Part print with two shaded views. Sizes in mm from the minimum x, y, z corner. A direction names the side the tool comes from. Round coordinates to 2 decimals unless told otherwise and drop trailing zeros. Order: outer loops, then holes, each group sorted by start corner. A loop starts at its lowest first (then second) coordinate and runs counter-clockwise, first axis right, second up. Notation, with made-up numbers: M -17,-24 L 34,-24 A30 ccw 34,13 Z; hole C 15.5,-22.75 d2. An arc over 180 degrees is marked long. Put each result on its own line as item: value.
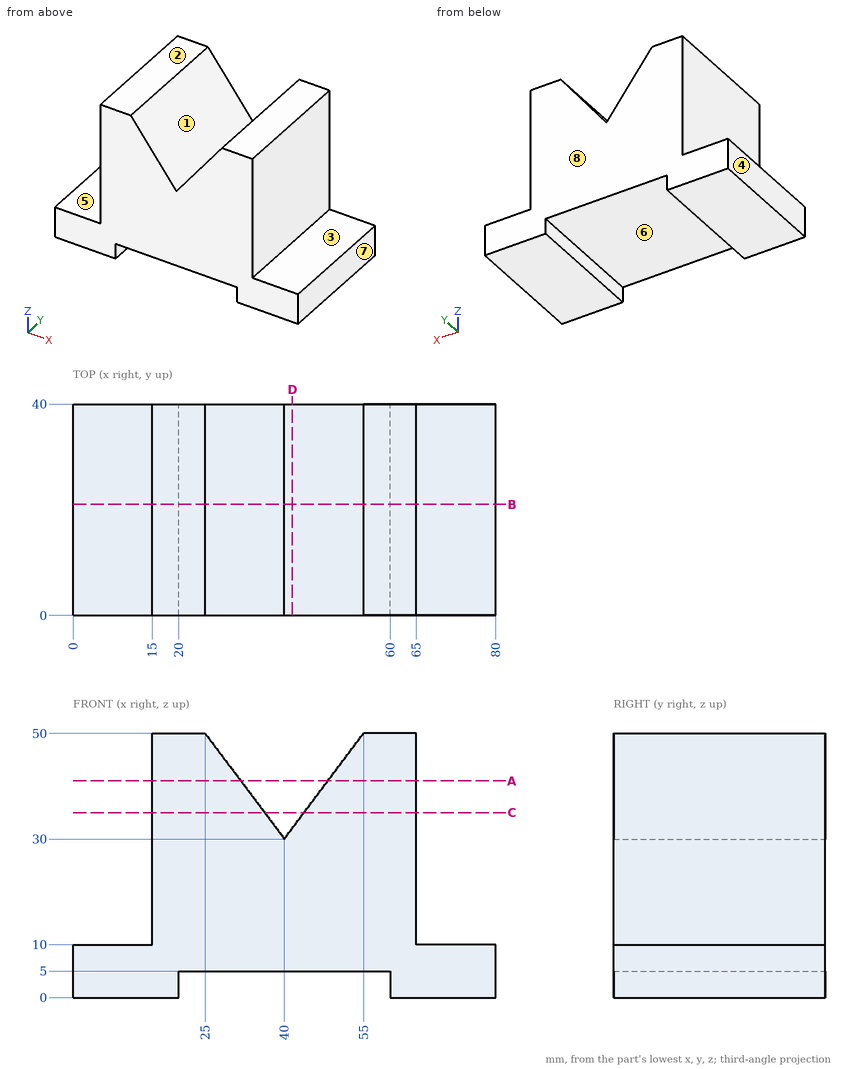
Item 1: Mould opens along X. For the marked faces 6, 7 and 8 say: pulls with the +X half, pulls with the -X half, needs draft (parallel to the pull), parting line crosses it, or undercut.
Answers below:
face 6: undercut
face 7: pulls with the +X half
face 8: needs draft
Item 2: Pin check, flat tips, straight feed: P1, Ø12, axis at x = 75, y = 11, coming from the +Z side; P2, Ø2, axis at y = 24.5, z = 15, coming from the +X side; P3, Ø5, axis at x = 37.5, y = 19.5, coming from the +Z side. Stop position of each tip, or through.
Answers below:
P1: z = 10
P2: x = 65
P3: z = 36.67
Item 3: Tool access for the marked faces 1, 2, 3, 4 and 5: list every direction of +Z, -Z, +X, -X, +Y, -Y with a clear straight run to the whole face (end or side of a thin tool).
Answers below:
face 1: +Z, +Y, -Y
face 2: +Z, +X, -X, +Y, -Y
face 3: +Z, +X, +Y, -Y
face 4: +Z, -Z, -X, +Y, -Y
face 5: +Z, -X, +Y, -Y
Item 4: Probe line 1 along X through (y, z) = (22.5, 17); line 2 along Z through (x, y) = (68, 7); line 3 along X through (y, z) = (7, 39). List the from-to ranges inside material, lowest first. Write a range as [from, to].
Answers below:
line 1: [15, 65]
line 2: [0, 10]
line 3: [15, 33.25], [46.75, 65]
Item 5: Band-saw the part on B-B on y = 21. Give the cut face in (x, z), and give its area (3 significant figures).
Answers below:
outline: M 0,0 L 20,0 L 20,5 L 60,5 L 60,0 L 80,0 L 80,10 L 65,10 L 65,50 L 55,50 L 40,30 L 25,50 L 15,50 L 15,10 L 0,10 Z
area: 2,300 mm²
Item 6: Band-saw the part on D-D on x = 41.5. Give the cut face in (y, z), and give its area (3 significant figures).
Answers below:
outline: M 0,5 L 40,5 L 40,32 L 0,32 Z
area: 1,080 mm²
Item 7: Band-saw the part on C-C on z = 35. Give the cut face in (x, y).
Answers below:
outline: M 15,0 L 36.25,0 L 36.25,40 L 15,40 Z; M 43.75,0 L 65,0 L 65,40 L 43.75,40 Z
Item 8: Band-saw the part on A-A on z = 41. Give the cut face in (x, y).
Answers below:
outline: M 15,0 L 31.75,0 L 31.75,40 L 15,40 Z; M 48.25,0 L 65,0 L 65,40 L 48.25,40 Z
